from build123d import *

# Parameters (mm, degrees)
BOSS_EXTRUDE1_DEPTH = 15.24
CUT_EXTRUDE1_DEPTH  = 19.05
CUT_EXTRUDE2_DEPTH  = 29.21
CUT_EXTRUDE4_REACH  = 35.15
SKETCH7_W           = 29.21
SKETCH7_H           = 19.05
FILLET3_R           = 2.54
FILLET6_R           = 0.762
FILLET7_R           = 2.286
FILLET9_R           = 3.175
FILLET10_R          = 0.762
FILLET11_R          = 0.635
FILLET12_R          = 0.254


with BuildPart() as part:
    # Sketch1 → Boss-Extrude1 (new, symmetric)
    with BuildSketch(Plane.XY):
        Polygon((-28.575, 0), (-28.575, 2), (-18.415, 2), (-18.415, 7.08), (13.335, 7.08), (13.335, 2), (28.575, 2), (28.575, 0), align=None)
    extrude(amount=BOSS_EXTRUDE1_DEPTH, both=True)

    # Sketch4 → Cut-Extrude1 (cut)
    with BuildSketch(Plane(origin=(0, 2, 0), x_dir=(1, 0, 0), z_dir=(0, 1, 0))):
        with BuildLine():
            Line((26.035, 11.43), (26.035, 8.89))
            ThreePointArc((26.035, 8.89), (24.13, 6.985), (22.225, 8.89))
            Line((22.225, 8.89), (22.225, 11.43))
            ThreePointArc((22.225, 11.43), (24.13, 13.335), (26.035, 11.43))
        make_face()
        with BuildLine():
            Line((26.035, -8.89), (26.035, -11.43))
            ThreePointArc((26.035, -11.43), (24.13, -13.335), (22.225, -11.43))
            Line((22.225, -11.43), (22.225, -8.89))
            ThreePointArc((22.225, -8.89), (24.13, -6.985), (26.035, -8.89))
        make_face()
        with BuildLine():
            Line((-22.225, 11.43), (-22.225, 8.89))
            ThreePointArc((-22.225, 8.89), (-24.13, 6.985), (-26.035, 8.89))
            Line((-26.035, 8.89), (-26.035, 11.43))
            ThreePointArc((-26.035, 11.43), (-24.13, 13.335), (-22.225, 11.43))
        make_face()
        with BuildLine():
            Line((-22.225, -8.89), (-22.225, -11.43))
            ThreePointArc((-22.225, -11.43), (-24.13, -13.335), (-26.035, -11.43))
            Line((-26.035, -11.43), (-26.035, -8.89))
            ThreePointArc((-26.035, -8.89), (-24.13, -6.985), (-22.225, -8.89))
        make_face()
    extrude(amount=-CUT_EXTRUDE1_DEPTH, mode=Mode.SUBTRACT)

    # Sketch5 → Cut-Extrude2 (cut)
    with BuildSketch(Plane(origin=(13.335, 0, 0), x_dir=(0, 0, -1), z_dir=(1, 0, 0))):
        Polygon((-12.3825, 2), (12.3825, 2), (12.3825, 6.445), (11.3665, 6.445), (11.3665, 7.08), (-11.3665, 7.08), (-11.3665, 6.445), (-12.3825, 6.445), align=None)
    extrude(amount=-CUT_EXTRUDE2_DEPTH, mode=Mode.SUBTRACT)

    # Sketch7 → Cut-Extrude4 (cut, up to next)
    with BuildSketch(Plane.XZ, mode=Mode.PRIVATE) as cut_extrude4_sk1:
        with Locations((0.635, 0)):
            Rectangle(SKETCH7_W, SKETCH7_H)
    cut_extrude4_tool1 = extrude(cut_extrude4_sk1.sketch, amount=-CUT_EXTRUDE4_REACH, mode=Mode.PRIVATE) & part.part
    add(cut_extrude4_tool1.solids().sort_by_distance((0.635, 0, 0))[0], mode=Mode.SUBTRACT)

    # Fillet3
    fillet3_edges = [part.edges().sort_by_distance(p)[0] for p in [
        (15.24, 1, 9.525),
        (15.24, 1, -9.525),
        (-13.97, 1, -9.525),
        (-13.97, 1, 9.525),
    ]]
    fillet(fillet3_edges, radius=FILLET3_R)

    # Fillet6
    fillet6_edges = [part.edges().sort_by_distance(p)[0] for p in [
        (13.335, 6.7625, -11.3665),
        (13.335, 6.7625, 11.3665),
    ]]
    fillet(fillet6_edges, radius=FILLET6_R)

    # Fillet7
    fillet7_edges = [part.edges().sort_by_distance(p)[0] for p in [
        (-15.875, 6.7625, 11.3665),
        (-15.875, 6.7625, -11.3665),
    ]]
    fillet(fillet7_edges, radius=FILLET7_R)

    # Fillet9
    fillet9_edges = [part.edges().sort_by_distance(p)[0] for p in [
        (28.575, 1, -15.24),
        (-28.575, 1, 15.24),
        (-28.575, 1, -15.24),
        (28.575, 1, 15.24),
    ]]
    fillet(fillet9_edges, radius=FILLET9_R)

    # Fillet10
    fillet10_edges = [part.edges().sort_by_distance(p)[0] for p in [
        (13.335, 2, -13.81125),
        (-18.415, 2, 0),
        (13.335, 2, 13.81125),
    ]]
    fillet(fillet10_edges, radius=FILLET10_R)

    # Fillet11
    fillet11_edges = [part.edges().sort_by_distance(p)[0] for p in [
        (-18.415, 7.08, 0),
        (-2.54, 7.08, 15.24),
        (19.7485, 2, 15.24),
        (-28.575, 2, 0),
        (-27.64506403, 2, -14.31006403),
        (-27.64506403, 2, 14.31006403),
        (19.7485, 2, -15.24),
        (28.575, 2, 0),
        (27.64506403, 2, -14.31006403),
        (27.64506403, 2, 14.31006403),
        (13.335, 4.921, 15.24),
        (13.335, 4.921, -15.24),
        (-22.2885, 2, 15.24),
        (-18.415, 4.921, 15.24),
        (-22.2885, 2, -15.24),
        (13.558184633, 2.223184633, 15.24),
        (13.558184633, 2.223184633, -15.24),
        (-18.638184633, 2.223184633, -15.24),
        (-18.638184633, 2.223184633, 15.24),
        (-18.415, 4.921, -15.24),
        (-2.54, 7.08, -15.24),
    ]]
    fillet(fillet11_edges, radius=FILLET11_R)

    # Fillet12
    fillet12_edges = [part.edges().sort_by_distance(p)[0] for p in [
        (-1.27, 6.445, -12.3825),
        (-1.27, 6.445, 12.3825),
    ]]
    fillet(fillet12_edges, radius=FILLET12_R)


solid = part.part
Could you check a few things on this model? Use its own coordinates, in mm. A direction names the side the tool comes from. Give positions to 0.01 mm unless a question says otherwise; leave off trailing zeros. Loops run counter-clockwise (first coordinate to the right, second up) from the corner with the lowest first, then second, coordinate; pieces in that order, holes last. Notation, with made-up numbers: (85.5, 16.25) -> (96.5, 16.25) arc R26 cw to (96.5, 41.25) -> close; hole circle Ø7 at (24.5, 29). An arc over 180 degrees is marked (long way). Return JSON: item names as keys, results as strings.
Item 1: If we section it at C-C on z = -3.5: List the corners of the cut face in (x, y) for me (3 decimals).
Geometry results:
{"outline": "(-28.575, 0) -> (-13.97, 0) -> (-13.97, 2) -> (-15.875, 2) -> (-15.875, 7.08) -> (-17.78, 7.08) arc R0.635 ccw to (-18.415, 6.445) -> (-18.415, 2.762) arc R0.762 cw to (-19.177, 2) -> (-27.94, 2) arc R0.635 ccw to (-28.575, 1.365) -> close; (15.24, 0) -> (28.575, 0) -> (28.575, 1.365) arc R0.635 ccw to (27.94, 2) -> (15.24, 2) -> close"}
Item 2: If we section it at D-D on y = 3.75: List the corners of the cut face in (x, z) for me (1 decimal).
Geometry results:
{"outline": "(-18.4, -14.6) arc R0.6 ccw to (-17.8, -15.2) -> (12.7, -15.2) arc R0.6 ccw to (13.3, -14.6) -> (13.3, -12.4) -> (-15.9, -12.4) -> (-15.9, 12.4) -> (13.3, 12.4) -> (13.3, 14.6) arc R0.6 ccw to (12.7, 15.2) -> (-17.8, 15.2) arc R0.6 ccw to (-18.4, 14.6) -> close"}
Item 3: If we section it at A-A on x = 24.13: List the corners of the cut face in (y, z) for me (3 decimals), plus the area to 3 significant figures.
Geometry results:
{"outline": "(0, -15.24) -> (1.365, -15.24) arc R0.635 ccw to (2, -14.605) -> (2, -13.335) -> (0, -13.335) -> close; (0, -6.985) -> (2, -6.985) -> (2, 6.985) -> (0, 6.985) -> close; (0, 13.335) -> (2, 13.335) -> (2, 14.605) arc R0.635 ccw to (1.365, 15.24) -> (0, 15.24) -> close", "area": "35.4 mm²"}
Item 4: Which directions (+Z, -Z, +X, -X, +Y, -Y) give clear straight access to the entire face, cutting with the end or side of a thin tool? Please do faces 4 (the cylindrical face through (-24.088, 1.014, -6.985)), 5 (the cylindrical face through (-15.2, 6.8, 10.7)), 6 (the flat face through (-1, 4, 12.382)).
Geometry results:
{"face 4": "+Y, -Y", "face 5": "+X, +Y", "face 6": "+X"}
Item 5: I need wall thicknesses on L1, parallel to Z at x = 11.5, y = 4.75; L2, parallel to X at y = 1.5, z = -11 (3 decimals); L3, parallel to X at y = 0.75, z = 2 (3 decimals). Which ranges of each line are inside material? Lowest first, please. Write a range as from..to.
Geometry results:
{"L1": "z = -15.24..-12.38, 12.38..15.24", "L2": "x = -28.56..-26.035, -22.225..22.225, 26.035..28.56", "L3": "x = -28.575..-13.97, 15.24..28.575"}
Item 6: I'm going to push flat-ended pins straight in: pin 1 (2.5 mm diameter, centred on y = 4, z = 14, fed in from +X); pin 2 (2 mm diameter, centred on x = -22.5, z = 5, fed in from +Y); pin 3 (1 mm diameter, centred on y = 3, z = -3, fed in from +X) (3 decimals). Where does each tip first touch, or does it pass through?
Geometry results:
{"pin 1": "stops at x = 13.34", "pin 2": "stops at y = 2", "pin 3": "stops at x = -15.875"}
Item 7: We'd pull the mould along Z, two halves only. Please class faces 1 (the cylindrical face through (27.67, 0.673, -14.285)), 2 (the cylindrical face through (-24.088, 1.014, 13.335)), 3 (the flat face through (-16.1, 7.08, 1.2)): +Z half, -Z half, draft (parallel to the pull), parting line (faces both ways), or undercut.
Geometry results:
{"face 1": "-Z half", "face 2": "undercut", "face 3": "draft"}
